Solid Edge part; units mm, degrees
sketch "Sketch1" plane through (0, 0, 0) normal (0, 0, 1) x (1, 0, 0)
  circle A0 centre (0, 0) radius 1.5
extrude "Protrusion1" add sketch "Sketch1" along normal blind 30
sketch "Sketch2" plane through (0, 0, 30) normal (0, 0, 1) x (1, 0, 0)
  circle A0 centre (0, 0) radius 3
extrude "ExtrudedProtrusion_2" add sketch "Sketch2" along normal blind 1.75
chamfer "Chamfer_1" distance 1.75 angle 45 1 edges at (-3, 0, 30)
sketch "Sketch3" plane through (0, 0, 31.75) normal (0, 0, 1) x (0, 1, 0)
  line L0 (0.8978, -1.555) -> (1.7956, 0)
  line L1 (1.7956, 0) -> (0.8978, 1.555)
  line L2 (0.8978, 1.555) -> (-0.8978, 1.555)
  line L3 (-0.8978, 1.555) -> (-1.7956, 0)
  line L4 (-1.7956, 0) -> (-0.8978, -1.555)
  line L5 (-0.8978, -1.555) -> (0.8978, -1.555)
extrude "ExtrudedCutout_1" cut sketch "Sketch3" against normal blind 1
sketch "Sketch4" plane through (0, 0, 0) normal (0, 0, -1) x (0, 1, 0)
  circle A0 centre (0, 0) radius 1.9215
extrude "ExtrudedCutout_2" cut sketch "Sketch4" against normal blind 11.75
properties material "Iron, grey cast type 20"
Model file for the job. Use its own axes, mm. A direction names the side the tool comes from. Round coordinates to 2 decimals unless told otherwise and drop trailing zeros. Loops run counter-clockwise (first coordinate to the right, second up) from the corner with the lowest first, then second, coordinate; pieces in that order, holes last. Notation, with made-up numbers: M 34,9 L 44,9 A24 ccw 44,25 Z; hole C 64,74.5 d7. An arc over 180 degrees is marked long. One line per question, with ' | ' between items.
1) Mould opens along Y. For faces 1 (the cylindrical face through (-1.5, -0.07, 20.87)), 2 (the flat face through (-0.79, -1.34, 31.26)), 3 (the flat face through (0, 0, 11.75)), 4 (the flat face through (-0.77, 1.35, 31.26)) say: +Y half, -Y half, draft (parallel to the pull), parting line (faces both ways), or undercut.
Solved:
face 1: parting line | face 2: undercut | face 3: draft | face 4: undercut
2) Drill centre lines: line 1 along Y through (x, z) = (-0.8, 30.5); line 2 along Z through (x, y) = (-0.55, -0.3); line 3 along X through (y, z) = (-0.2, 14.75). Where is each one in solid material? Low to high.
Solved:
line 1: y = -1.56 to 1.56 | line 2: z = 11.75 to 30.75 | line 3: x = -1.49 to 1.49
3) Band-saw the part on A-A (y = 0). Give the cut face in (x, z) (3 decimals), then the cut area to 3 significant figures.
Solved:
outline: M -3,31.75 L -1.5,30.25 L -1.5,11.75 L 1.5,11.75 L 1.5,30.25 L 3,31.75 L 1.555,31.75 L 1.555,30.75 L -1.555,30.75 L -1.555,31.75 Z | area: 59.1 mm²
4) Band-saw the part on B-B (z = 22.75). Give the cut face in (x, y), then the cut area to 3 significant figures.
Solved:
outline: C 0,0 d3 | area: 7.07 mm²
5) Flat gauge pins, fed straight in: pin 1 (0.9 mm diameter, centred on x = -0.5, y = 0.5, fed in from +Z); pin 2 (1 mm diameter, centred on y = -1.5, z = 23, fed in from -X); pin 3 (2 mm diameter, centred on x = -2, z = 16.5, fed in from -Y). Where does each tip first touch, or does it go through?
Solved:
pin 1: stops at z = 30.75 | pin 2: stops at x = -1.12 | pin 3: stops at y = -1.12
6) 3-axis set-ups, long thin cutter, end or side, ignore diameter. For faces 5 (the flat face through (-1.555, 0, 31)), 6 (the flat face through (1.3, -1.3, 31.75)): which of +Z, -Z, +X, -X, +Y, -Y reach the whole face in a straight line?
Solved:
face 5: +Z | face 6: +Z, +X, -X, +Y, -Y
